from build123d import *

# Parameters (mm, degrees)
F1_DEPTH      = 230.1875
F2_W          = 19.05
F2_H          = 9.525
F3_DEPTH      = 493
F3_DEPTH_BACK = 57.151


# Not quite as in the source:
# - an extrude ends at something that could not be found from the text; its depth is read off the source's solid


with BuildPart() as f1:
    # F0 (on Right) → F1 (new body, symmetric)
    with BuildSketch(Plane.YZ):
        Polygon((-19.05, 57.15), (-19.05, 0), (0, 0), (0, 38.1), (-6.35, 38.1), (-6.35, 57.15), align=None)
    extrude(amount=F1_DEPTH, both=True)

    # F2 (on Top) → F3 (cut, two sides)
    with BuildSketch(Plane.XY) as f3_sk:
        with Locations((220.6625, -4.7625)):
            Rectangle(F2_W, F2_H)
        with Locations((-220.6625, -4.7625)):
            Rectangle(F2_W, F2_H)
    extrude(amount=-F3_DEPTH, mode=Mode.SUBTRACT)
    extrude(f3_sk.sketch, amount=F3_DEPTH_BACK, mode=Mode.SUBTRACT)


solid = f1.part
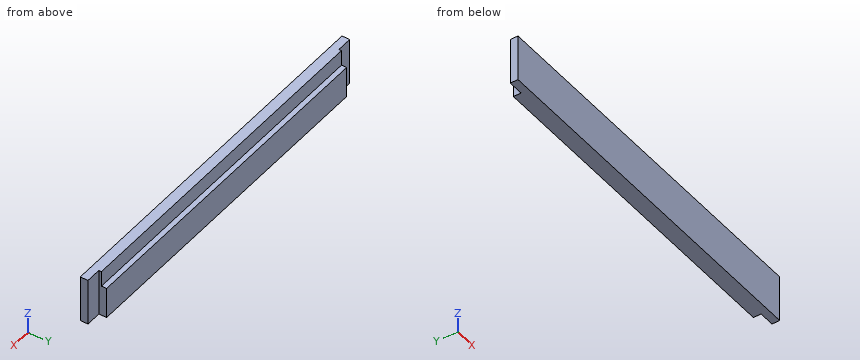
Can you work these out from the model? Positions are in its coordinate system, mm. Round coordinates to 2 decimals unless told otherwise and drop trailing zeros. Write each loop counter-clockwise with the first axis right and the second up, starting at its lowest first coordinate (ties: lowest second). Pieces come first, ordered by that corner, then holes. Notation, with made-up numbers: (54, -17.75) -> (80, -17.75) arc R28 cw to (80, 21.25) -> close; hole circle Ø2 at (36, 9.25). An arc over 180 degrees is marked (long way). Use one line per item in the form item = value. Start each with the question number.
Q1. I'm going to push flat-ended pins straight in: P1, Ø9.5, axis at x = -220.5, z = 30, coming from the +Y side (3 decimals); P2, Ø1, axis at x = 134, y = -2.5, coming from the +Z side; P3, Ø5, axis at y = -4, z = 25, coming from the +X side. Where does each tip first touch, or does it pass through?
Q2. If I drill on probe 1 along Z at (x, y) = (-108, -4.75); probe 2 along X at (y, z) = (-5.5, 22.5); probe 3 along Y at (x, z) = (-134.5, 48), over which ranges is the centre line in solid material (lowest first)? Write a range as [from, to].
Q3. Imagine slicing it at B-B (x = -149). Please give me the cut outline in (y, z).
Worked out:
q1.P1 = -9.525
q1.P2 = 38.1
q1.P3 = 211.14
q2.probe_1 = [0, 38.1]
q2.probe_2 = [-211.14, 211.14]
q2.probe_3 = [-19.05, -6.35]
q3.outline = (-19.05, 0) -> (0, 0) -> (0, 38.1) -> (-6.35, 38.1) -> (-6.35, 57.15) -> (-19.05, 57.15) -> close
